```python
from build123d import *

# Parameters (mm, degrees)
F0_R      = 11.43
F1_DEPTH  = 6.35
F2_R      = 3.4925
F3_DEPTH  = 3.81
F4_R      = 5.715
F4_R_2    = 4.7625
F5_DEPTH  = 3.81
F7_DEPTH  = 3.81
F8_R      = 3.81
F9_DEPTH  = 3.175
F10_R     = 1.778
F11_DEPTH = 0.635


with BuildPart() as f1:
    # F0 (on Front) → F1 (new body)
    with BuildSketch(Plane.XZ):
        Circle(F0_R)
    extrude(amount=F1_DEPTH)

    # F2 (on face) → F3 (cut)
    with BuildSketch(Plane.XZ.offset(6.35)):
        Circle(F2_R)
    extrude(amount=-F3_DEPTH, mode=Mode.SUBTRACT)

    # F4 (on face) → F5 (cut)
    with BuildSketch(Plane.XZ.offset(6.35)):
        Circle(F4_R)
        Circle(F4_R_2, mode=Mode.SUBTRACT)
    extrude(amount=-F5_DEPTH, mode=Mode.SUBTRACT)

    # F6 (on face) → F7 (cut)
    with BuildSketch(Plane.XZ.offset(6.35)):
        with BuildLine():
            Line((0.3175, 3.4780382402), (0.3175, 4.4336462139))
            ThreePointArc((0.3175, 4.4336462139), (0, 4.445), (-0.3175, 4.4336462139))
            Line((-0.3175, 4.4336462139), (-0.3175, 3.4780382402))
            ThreePointArc((-0.3175, 3.4780382402), (0, 3.4925), (0.3175, 3.4780382402))
        make_face()
        with BuildLine():
            Line((-3.4780382402, 0.3175), (-4.4336462139, 0.3175))
            ThreePointArc((-4.4336462139, 0.3175), (-4.445, 0), (-4.4336462139, -0.3175))
            Line((-4.4336462139, -0.3175), (-3.4780382402, -0.3175))
            ThreePointArc((-3.4780382402, -0.3175), (-3.4925, 0), (-3.4780382402, 0.3175))
        make_face()
        with BuildLine():
            ThreePointArc((4.4336462139, -0.3175), (4.4421606466, -0.1588514703), (4.445, 0))
            ThreePointArc((4.445, 0), (4.4421606466, 0.1588514703), (4.4336462139, 0.3175))
            Line((4.4336462139, 0.3175), (3.4780382402, 0.3175))
            ThreePointArc((3.4780382402, 0.3175), (3.4888826867, 0.1589145938), (3.4925, 0))
            ThreePointArc((3.4925, 0), (3.4888826867, -0.1589145938), (3.4780382402, -0.3175))
            Line((3.4780382402, -0.3175), (4.4336462139, -0.3175))
        make_face()
        with BuildLine():
            ThreePointArc((-0.3175, -4.4336462139), (0, -4.445), (0.3175, -4.4336462139))
            Line((0.3175, -4.4336462139), (0.3175, -3.4780382402))
            ThreePointArc((0.3175, -3.4780382402), (0, -3.4925), (-0.3175, -3.4780382402))
            Line((-0.3175, -3.4780382402), (-0.3175, -4.4336462139))
        make_face()
        with BuildLine():
            ThreePointArc((-0.3175, 4.4336462139), (0, 4.445), (0.3175, 4.4336462139))
            Line((0.3175, 4.4336462139), (0.3175, 4.7519048812))
            ThreePointArc((0.3175, 4.7519048812), (0.1588383664, 4.7598504833), (0, 4.7625))
            ThreePointArc((0, 4.7625), (-0.1588383664, 4.7598504833), (-0.3175, 4.7519048812))
            Line((-0.3175, 4.7519048812), (-0.3175, 4.4336462139))
        make_face()
        with BuildLine():
            ThreePointArc((-4.4336462139, -0.3175), (-4.445, 0), (-4.4336462139, 0.3175))
            Line((-4.4336462139, 0.3175), (-4.7519048812, 0.3175))
            ThreePointArc((-4.7519048812, 0.3175), (-4.7598504833, 0.1588383664), (-4.7625, 0))
            ThreePointArc((-4.7625, 0), (-4.7598504833, -0.1588383664), (-4.7519048812, -0.3175))
            Line((-4.7519048812, -0.3175), (-4.4336462139, -0.3175))
        make_face()
        with BuildLine():
            ThreePointArc((4.4336462139, 0.3175), (4.4421606466, 0.1588514703), (4.445, 0))
            ThreePointArc((4.445, 0), (4.4421606466, -0.1588514703), (4.4336462139, -0.3175))
            Line((4.4336462139, -0.3175), (4.7519048812, -0.3175))
            ThreePointArc((4.7519048812, -0.3175), (4.7598504833, -0.1588383664), (4.7625, 0))
            ThreePointArc((4.7625, 0), (4.7598504833, 0.1588383664), (4.7519048812, 0.3175))
            Line((4.7519048812, 0.3175), (4.4336462139, 0.3175))
        make_face()
        with BuildLine():
            Line((0.3175, -4.7519048812), (0.3175, -4.4336462139))
            ThreePointArc((0.3175, -4.4336462139), (0, -4.445), (-0.3175, -4.4336462139))
            Line((-0.3175, -4.4336462139), (-0.3175, -4.7519048812))
            ThreePointArc((-0.3175, -4.7519048812), (-0.1588383664, -4.7598504833), (0, -4.7625))
            ThreePointArc((0, -4.7625), (0.1588383664, -4.7598504833), (0.3175, -4.7519048812))
        make_face()
    extrude(amount=-F7_DEPTH, mode=Mode.SUBTRACT)

    # F8 (on face) → F9 (cut)
    with BuildSketch(Plane.XZ.offset(2.54)):
        Circle(F8_R)
    extrude(amount=F9_DEPTH, mode=Mode.SUBTRACT)

    # F10
    f10_edges = [f1.edges().sort_by_distance(p)[0] for p in [
        (-11.43, -6.35, 0),
        (-11.43, 0, 0),
    ]]
    fillet(f10_edges, radius=F10_R)

    # F8 (on face) → F11 (join)
    with BuildSketch(Plane.XZ.offset(2.54)):
        with BuildLine():
            ThreePointArc((0.3175, -3.7967477859), (2.6940768363, -2.6940768363), (3.7967477859, -0.3175))
            Line((3.7967477859, -0.3175), (3.4780382402, -0.3175))
            ThreePointArc((3.4780382402, -0.3175), (2.4695704333, -2.4695704333), (0.3175, -3.4780382402))
            Line((0.3175, -3.4780382402), (0.3175, -3.7967477859))
        make_face()
        with BuildLine():
            Line((3.4780382402, 0.3175), (3.7967477859, 0.3175))
            ThreePointArc((3.7967477859, 0.3175), (2.6940768363, 2.6940768363), (0.3175, 3.7967477859))
            Line((0.3175, 3.7967477859), (0.3175, 3.4780382402))
            ThreePointArc((0.3175, 3.4780382402), (2.4695704333, 2.4695704333), (3.4780382402, 0.3175))
        make_face()
        with BuildLine():
            Line((-0.3175, 3.4780382402), (-0.3175, 3.7967477859))
            ThreePointArc((-0.3175, 3.7967477859), (-2.6940768363, 2.6940768363), (-3.7967477859, 0.3175))
            Line((-3.7967477859, 0.3175), (-3.4780382402, 0.3175))
            ThreePointArc((-3.4780382402, 0.3175), (-2.4695704333, 2.4695704333), (-0.3175, 3.4780382402))
        make_face()
        with BuildLine():
            ThreePointArc((-3.7967477859, -0.3175), (-2.6940768363, -2.6940768363), (-0.3175, -3.7967477859))
            Line((-0.3175, -3.7967477859), (-0.3175, -3.4780382402))
            ThreePointArc((-0.3175, -3.4780382402), (-2.4695704333, -2.4695704333), (-3.4780382402, -0.3175))
            Line((-3.4780382402, -0.3175), (-3.7967477859, -0.3175))
        make_face()
    extrude(amount=F11_DEPTH)


solid = f1.part
```
For this review, take the finished solid that the model builds, in its own axes (mm). A direction names the side the tool comes from. Round coordinates to 2 decimals unless told otherwise and drop trailing zeros. Write each loop counter-clockwise with the first axis right and the second up, starting at its lowest first coordinate (ties: lowest second). Pieces come first, ordered by that corner, then holes.
1) Machinability: for faces 1 (the face through (-3, -6.35, 3)), 2 (the face through (5.45, -4.47, 1.72)), 3 (the face through (-2.58, -5.715, 2.58)), which of the approach directions +Z, -Z, +X, -X, +Y, -Y give a long, thin tool a straight path to every point of the face, cutting with its end or side? Answer none if there is none.
Answer below:
face 1: +Z, -Z, +X, -X, -Y
face 2: -Y
face 3: none
2) Take a section at B-B on x = 0. Give the boundary of the cut face in (y, z) (3 decimals).
Answer below:
outline: (-6.35, -9.652) arc R1.778 ccw to (-4.572, -11.43) - (-1.778, -11.43) arc R1.778 ccw to (0, -9.652) - (0, 9.652) arc R1.778 ccw to (-1.778, 11.43) - (-4.572, 11.43) arc R1.778 ccw to (-6.35, 9.652) - (-6.35, 5.715) - (-2.54, 5.715) - (-2.54, -5.715) - (-6.35, -5.715) - close
3) Mouldability with a two-part tool opening along Z and no side actions: class faces 4 (the face through (3, -6.35, 3)), 5 (the face through (3.401, -4.472, 3.334)) as +Z half, -Z half, draft (parallel to the pull), parting line (faces both ways), or undercut.
Answer below:
face 4: draft
face 5: undercut
4) Take a section at A-A on y = -6. Give the boundary of the cut face in (x, z) (1 decimal).
Answer below:
outline: circle Ø21.4 at (0, 0); (-4.8, -0.3) arc R4.8 ccw to (-0.3, -4.8) - (-0.3, -3.5) arc R3.5 cw to (-3.5, -0.3) - close; (-4.8, 0.3) - (-3.5, 0.3) arc R3.5 cw to (-0.3, 3.5) - (-0.3, 4.8) arc R4.8 ccw to start; (0.3, -4.8) arc R4.8 ccw to (4.8, -0.3) - (3.5, -0.3) arc R3.5 cw to (0.3, -3.5) - close; (0.3, 3.5) arc R3.5 cw to (3.5, 0.3) - (4.8, 0.3) arc R4.8 ccw to (0.3, 4.8) - close; hole circle Ø11.4 at (0, 0)
5) For line 1 along Z through (x, y) = (0, -4.3) (3 decimals); line 2 along X through (y, z) = (-4.25, -0.5); line 3 along X through (y, z) = (-4.5, -5), list the stretches that pass through material, from the lowest coordinate up.
Answer below:
line 1: z = -11.43 to -5.715, 5.715 to 11.43
line 2: x = -11.42 to -5.69, -4.74 to -3.78, 3.78 to 4.74, 5.69 to 11.42
line 3: x = -10.28 to -2.77, 2.77 to 10.28
6) Take a section at D-D on y = -1.5. Give the boundary of the cut face in (x, z), then the cut area to 3 significant figures.
Answer below:
outline: circle Ø22.82 at (0, 0)
area: 409 mm2
7) Take a section at C-C on z = 0. Give the boundary of the cut face in (x, y) (3 decimals), then the cut area to 3 significant figures.
Answer below:
outline: (-11.43, -4.572) arc R1.778 ccw to (-9.652, -6.35) - (-5.715, -6.35) - (-5.715, -2.54) - (5.715, -2.54) - (5.715, -6.35) - (9.652, -6.35) arc R1.778 ccw to (11.43, -4.572) - (11.43, -1.778) arc R1.778 ccw to (9.652, 0) - (-9.652, 0) arc R1.778 ccw to (-11.43, -1.778) - close
area: 98.9 mm2
8) Insertion check: pin 1 Ø1.5 at (y, z) = (-0.5, -7.5) entering from -X; pin 2 Ø1.5 at (y, z) = (-4.5, 4.5) entering from +X; pin 3 Ø1 at (x, y) = (-4, -4) entering from -Z. Each pin has a flat end and moves straight along its axis. Give the tip position at first contact, or say it passes through.
Answer below:
pin 1: stops at x = -8.86
pin 2: stops at x = 10.8
pin 3: stops at z = -10.88
